Geometry: final body of the model. Coordinates: model frame, mm. A direction names the side the tool comes from. Round coordinates to 2 decimals unless told otherwise and drop trailing zeros. Loops run counter-clockwise (first coordinate to the right, second up) from the corner with the lowest first, then second, coordinate; pieces in that order, holes last. Notation, with made-up numbers: M 77.25,61.25 L 123.25,61.25 A35 cw 123.25,95.25 Z; hole C 25,-39 d2. An arc over 180 degrees is marked long. Return JSON: item names as keys, results as strings.
Autodesk Inventor part; units mm, degrees
ref_plane "YZ Plane" through (0, 0, 0) normal (1, 0, 0) x (0, 1, 0)
ref_plane "XZ Plane" through (0, 0, 0) normal (0, 1, 0) x (-1, 0, 0)
ref_plane "XY Plane" through (0, 0, 0) normal (0, 0, 1) x (1, 0, 0)
sketch "Эскиз1" plane through (0, 0, 0) normal (0, 1, 0) x (-1, 0, 0)
  line L0 (0, 0) -> (-8, 0)
  line L1 (-8, 0) -> (-8, -37)
  line L2 (-8, -37) -> (0, -37)
  line L3 (0, -37) -> (0, 0)
  circle A0 centre (-8, 0) radius 1.6
  line L4 (-8, -37) -> (-2, -37)
  line L5 (-2, -37) -> (-2, -41)
  line L6 (-2, -41) -> (-14, -41)
  line L7 (-14, -41) -> (-14, 4)
  line L8 (-14, 4) -> (0, 4)
  line L9 (0, 4) -> (0, 0)
  line L10 (-2, -41) -> (0, -41)
  line L11 (0, -41) -> (0, -37)
  line L12 (0, 4) -> (4, 4)
  line L13 (4, 4) -> (4, -41)
  line L14 (4, -41) -> (0, -41)
  line L15 (0, -41) -> (0, 4)
  line L16 (4, 4) -> (4, -2)
  line L17 (4, -2) -> (-2, -2)
  line L18 (-2, -2) -> (-2, -37)
  line L19 (4, -41) -> (4, -35)
  line L20 (4, -35) -> (-2, -35)
  circle A1 centre (-8, -37) radius 1.6
  dimension "d0" = 8
  dimension "d1" = 37
  dimension "d2" = 3.2
  dimension "d4" = 6
  dimension "d5" = 4
  dimension "d6" = 12
  dimension "d7" = 45
  dimension "d10" = 4
  dimension "d13" = 6
  dimension "d14" = 6
  dimension "d15" = 6
  dimension "d28" = 3.2
extrude "Выдавливание1" add sketch "Эскиз1" along normal blind 6 contours L3 L17 L18 L2 A1 L1 A0 L0 | L9 L12 L13 L17 L3 | L0 A0 L1 A1 L2 L5 L6 L7 L8 L9 | L20 L13 L14 L11 L3 | L3 L2 L18 L20 | L11 L10 L5 L2
sketch "Эскиз3" plane through (-4, 0, 4) normal (0, 0, 1) x (1, 0, 0)
  line L0 (0, 0) -> (18, 0)
  line L1 (0, 0) -> (4, 0)
  line L2 (4, 0) -> (4, 3)
  line L3 (4, 3) -> (0, 3)
  line L4 (0, 3) -> (0, 0)
  circle A0 centre (4, 3) radius 1.6
  dimension "d16" = 4
  dimension "d17" = 3
  dimension "d18" = 3.2
extrude "Выдавливание2" cut sketch "Эскиз3" against normal blind 45 contours A0 L3 L2 | L2 L3 A0
fillet "Сопряжение2" radius 2 5 edges at (-4, 6, 1) (-4, 6, -38) (-4, 0, -38) (-4, 0, 1) (14, 6, -18.5)
sketch "Эскиз5" plane through (2, 0, -2) normal (0, 0, -1) x (-1, 0, 0)
  line L0 (0, 0) -> (0, 6)
  line L1 (0, 0) -> (6.2917, 0) construction
  line L2 (0, 0) -> (-3.4641, 6)
  line L3 (-10, 6) -> (4, 6)
  line L4 (0, 0) -> (6.9282, 0) construction
  line L5 (0, 6) -> (-3, 6)
  line L6 (-3, 6) -> (0, 0)
  line L7 (0, 0) -> (0, 6)
  point P0 (2, 0)
  dimension "d24" = 120
  dimension "d25" = 3
extrude "Выдавливание3" cut sketch "Эскиз5" along normal blind 33 contours L6 L3 L0
properties part number "krepleniye"
Q1. Pull-direction query (Y, two-part tool) for faces 3 (the cylindrical face through (13.43, 5.4, -18.18)), 4 (the cylindrical face through (-0.35, 1.44, -37.96)), 5 (the flat face through (14, 2, -19)); classes: pulls with the +Y half, pulls with the -Y half, needs draft (parallel to the pull), parting line crosses it, or undercut.
Determined:
{"face 3": "pulls with the +Y half", "face 4": "undercut", "face 5": "needs draft"}
Q2. Pin query (flat end, axial travel): pin 1 (1 mm diameter, centred on y = 5, z = -9.5, fed in from -X). Return the tip coordinate at first contact, or that it passes through.
Determined:
{"pin 1": "stops at x = 4.25"}
Q3. Section query B-B (x = 8). Output: boundary loops of the cut face in (y, z), plus the area to 3 significant figures.
Determined:
{"outline": "M 0,-41 L 6,-41 L 6,-38.6 L 0,-38.6 Z; M 0,-35.4 L 6,-35.4 L 6,-1.6 L 0,-1.6 Z; M 0,1.6 L 6,1.6 L 6,4 L 0,4 Z", "area": "232 mm^2"}
Q4. Section query C-C (z = -37). Output: boundary loops of the cut face in (x, y).
Determined:
{"outline": "M -4,2 A2 ccw -2,0 L 6.4,0 L 6.4,6 L -2,6 A2 ccw -4,4 Z; M 9.6,0 L 14,0 L 14,4 A2 ccw 12,6 L 9.6,6 Z; hole C 0,3 d3.2"}
Q5. Section query A-A (y = 3). Output: boundary loops of the cut face in (x, z), plus the area to 3 significant figures.
Determined:
{"outline": "M -4,-41 L -1.6,-41 L -1.6,-35 L -4,-35 Z; M -4,-2 L -1.6,-2 L -1.6,4 L -4,4 Z; M 1.6,-41 L 14,-41 L 14,4 L 1.6,4 L 1.6,-2 L 3.5,-2 L 3.5,-35 L 1.6,-35 Z; hole C 8,-37 d3.2; hole C 8,0 d3.2", "area": "508 mm^2"}
Q6. Section query D-D (x = 0). Output: boundary loops of the cut face in (y, z).
Determined:
{"outline": "M 0,-41 L 1.4,-41 L 1.4,-35 L 0,-35 Z; M 0,-2 L 1.4,-2 L 1.4,4 L 0,4 Z; M 4.6,-41 L 6,-41 L 6,-35 L 4.6,-35 Z; M 4.6,-2 L 6,-2 L 6,4 L 4.6,4 Z"}
Q7. Material intervals for L1, parallel to Z at x = 8, y = 4.55; L2, parallel to Y at x = 0, z = -39.15; L3, parallel to X at y = 1.85, z = -37, sorted ascending.
Determined:
{"L1": "z = -41 to -38.6, -35.4 to -1.6, 1.6 to 4", "L2": "y = 0 to 1.4, 4.6 to 6", "L3": "x = -3.99 to -1.11, 1.11 to 6.4, 9.6 to 14"}
Q8. Reachability of faces 1 (the flat face through (-2, 4, -35)), 2 (the cylindrical face through (-0.35, 1.44, 1.04)) from +Z, -Z, +X, -X, +Y, -Y: full face, straight path, thin tool, end or side. Return the list, or none.
Determined:
{"face 1": "-X, +Y", "face 2": "+Z, -Z"}
